Could you check a few things on this model? Use its own coordinates, in mm. A direction names the side the tool comes from. Round coordinates to 2 decimals unless told otherwise and drop trailing zeros. Loops run counter-clockwise (first coordinate to the right, second up) from the corner with the lowest first, then second, coordinate; pieces in that order, holes last. Notation, with made-up numbers: (-32.5, -38) -> (-0.5, -38) arc R12 ccw to (-0.5, -16) -> close; hole circle Ø8 at (28, -17). An arc over 180 degrees is marked (long way). One line per item, written item: value.
```python
from build123d import *

# Parameters (mm, degrees)
SKETCH_2_W          = 40
SKETCH_2_H          = 40
EXTRUDE_2_DEPTH     = 3
SKETCH_3_R          = 2
SKETCH_3_R_2        = 5.125
SKETCH_3_W          = 3
SKETCH_3_H          = 12
CUT_EXTRUDE_1_DEPTH = 3
EXTRUDE_START       = 20
SKETCH_9_W          = 40
SKETCH_9_H          = 40
EXTRUDE_4_DEPTH     = 3
SKETCH_3_3_R        = 2
EXTRUDE_5_DEPTH     = 24
EXTRUDE_START_2     = -2
SKETCH_2_8_R        = 2
EXTRUDE_6_DEPTH     = 2


with BuildPart() as part:
    # Sketch 2 → Extrude 2 (new body)
    with BuildSketch(Plane(origin=(0, 0, 0), x_dir=(1, 0, 0), z_dir=(0, 1, 0))):
        Rectangle(SKETCH_2_W, SKETCH_2_H)
    extrude(amount=EXTRUDE_2_DEPTH)

    # Sketch 3 → Cut-Extrude 1 (cut)
    with BuildSketch(Plane(origin=(0, 0, 0), x_dir=(1, 0, 0), z_dir=(0, 1, 0))):
        with Locations(Location((-15.224798987, -15.224798987, 0), (0, 0, 270))):
            Circle(SKETCH_3_R)
        with Locations(Location((15.224798987, -15.224798987, 0), (0, 0, 270))):
            Circle(SKETCH_3_R)
        with Locations(Location((15.224798987, 15.224798987, 0), (0, 0, 270))):
            Circle(SKETCH_3_R)
        with Locations(Location((-15.224798987, 15.224798987, 0), (0, 0, 270))):
            Circle(SKETCH_3_R)
        with Locations(Location((-7, 0, 0), (0, 0, 270))):
            Circle(SKETCH_3_R_2)
        with Locations((9.5, 0.011605537)):
            Rectangle(SKETCH_3_W, SKETCH_3_H)
    extrude(amount=CUT_EXTRUDE_1_DEPTH, mode=Mode.SUBTRACT)



with BuildPart() as body_2:
    # Sketch 9 → Extrude 4 (new body)
    with BuildSketch(Plane(origin=(0, 3, 0), x_dir=(1, 0, 0), z_dir=(0, 1, 0)).offset(EXTRUDE_START)):
        Rectangle(SKETCH_9_W, SKETCH_9_H)
    extrude(amount=EXTRUDE_4_DEPTH)

    # Sketch 3_3 → Extrude 5 (add)
    with BuildSketch(Plane(origin=(0, 0, 0), x_dir=(1, 0, 0), z_dir=(0, 1, 0))):
        with Locations(Location((-15.224798987, -15.224798987, 0), (0, 0, 270))):
            Circle(SKETCH_3_3_R)
        with Locations(Location((15.224798987, -15.224798987, 0), (0, 0, 270))):
            Circle(SKETCH_3_3_R)
        with Locations(Location((15.224798987, 15.224798987, 0), (0, 0, 270))):
            Circle(SKETCH_3_3_R)
        with Locations(Location((-15.224798987, 15.224798987, 0), (0, 0, 270))):
            Circle(SKETCH_3_3_R)
    extrude(amount=EXTRUDE_5_DEPTH)


with BuildPart() as part_1:
    add(part.part)

    add(body_2.part)  # Extrude 6 merges body 2
    # Sketch 2_8 → Extrude 6 (add)
    with BuildSketch(Plane(origin=(0, 0, 0), x_dir=(1, 0, 0), z_dir=(0, 1, 0)).offset(EXTRUDE_START_2)):
        with Locations(Location((15.224798987, 15.224798987, 0), (0, 0, 270))):
            Circle(SKETCH_2_8_R)
        with Locations(Location((-15.224798987, -15.224798987, 0), (0, 0, 270))):
            Circle(SKETCH_2_8_R)
        with Locations(Location((15.224798987, -15.224798987, 0), (0, 0, 270))):
            Circle(SKETCH_2_8_R)
        with Locations(Location((-15.224798987, 15.224798987, 0), (0, 0, 270))):
            Circle(SKETCH_2_8_R)
    extrude(amount=EXTRUDE_6_DEPTH)


solid = part_1.part
```
(1) Imagine slicing it at D-D on z = -18. Write out the boundary of the cut face in (x, y), then the cut area to 3 significant figures.
Results below:
outline: (-20, 0) -> (20, 0) -> (20, 3) -> (-20, 3) -> close; (-20, 23) -> (20, 23) -> (20, 26) -> (-20, 26) -> close
area: 240 mm²
(2) For pin 1 Ø4 at (x, y) = (-10.5, 16) entering from +Z; pin 2 Ø1.5 at (x, z) = (14.5, -10.5) entering from -Y, each with a flat end and sliding along its axis, tell me the tip position at first contact or that it passes through.
Results below:
pin 1: passes through
pin 2: stops at y = 0
(3) On a 3-axis mill with a long thin cutter (end or side, diameter ignored), from which of +Z, -Z, +X, -X, +Y, -Y can I reach the whole of each face in a straight line? I mean faces 4 (the face through (-15, -2, 15)), 5 (the face through (-13.242, -1.014, 14.964)), 6 (the face through (-13.873, 12.86, -16.699)). Say none if no direction works.
Results below:
face 4: +Z, -Z, +X, -X, -Y
face 5: -Y
face 6: none
(4) Imagine slicing it at B-B on x = -7. Write out the boundary of the cut face in (y, z) (3 decimals), then the cut area to 3 significant figures.
Results below:
outline: (0, -20) -> (3, -20) -> (3, -5.125) -> (0, -5.125) -> close; (0, 5.125) -> (3, 5.125) -> (3, 20) -> (0, 20) -> close; (23, -20) -> (26, -20) -> (26, 20) -> (23, 20) -> close
area: 209 mm²
(5) Imagine slicing it at A-A on z = 0. Write out the boundary of the cut face in (x, y) (3 decimals), then the cut area to 3 significant figures.
Results below:
outline: (-20, 0) -> (-12.125, 0) -> (-12.125, 3) -> (-20, 3) -> close; (-20, 23) -> (20, 23) -> (20, 26) -> (-20, 26) -> close; (-1.875, 0) -> (8, 0) -> (8, 3) -> (-1.875, 3) -> close; (11, 0) -> (20, 0) -> (20, 3) -> (11, 3) -> close
area: 200 mm²
(6) Imagine slicing it at C-C on x = 2.5. Write out the boundary of the cut face in (y, z).
Results below:
outline: (0, -20) -> (3, -20) -> (3, 20) -> (0, 20) -> close; (23, -20) -> (26, -20) -> (26, 20) -> (23, 20) -> close
(7) We'd pull the mould along Y, two halves only. Please class faces 1 (the face through (0, 26, 0)), 2 (the face through (-13.242, 12.86, 14.964)), 3 (the face through (17.208, -1.014, 14.964)): +Y half, -Y half, draft (parallel to the pull), parting line (faces both ways), or undercut.
Results below:
face 1: +Y half
face 2: undercut
face 3: draft
(8) Please list where these lines run through material, in increasing order: L1, parallel to Y at x = 1, z = 10; L2, parallel to X at y = 4.75, z = 15; L3, parallel to X at y = 0.5, z = 4.
Results below:
L1: y = 0 to 3, 23 to 26
L2: x = -17.21 to -13.24, 13.24 to 17.21
L3: x = -20 to -10.2, -3.8 to 8, 11 to 20
